```python
from build123d import *

# Parameters (mm, degrees)
SKETCH_W             = 140
SKETCH_H             = 102
PAD_DEPTH            = 30
SKETCH001_W          = 56.560638
SKETCH001_H          = 58.617586
SKETCH001_W_2        = 18.878723
SKETCH001_W_3        = 44
SKETCH001_H_2        = 35.382414
POCKET_DEPTH         = 28
FILLET_R             = 5
SKETCH002_W          = 65
SKETCH002_H          = 90
POCKET001_DEPTH      = 8
FILLET001_R          = 2
BODY_PLACEMENT_ANGLE = 90


with BuildPart() as part:
    # Sketch → Pad (new body)
    with BuildSketch(Plane.XY):
        Rectangle(SKETCH_W, SKETCH_H)
    extrude(amount=PAD_DEPTH)

    # Sketch001 (on DatumPlane) → Pocket (cut)
    with BuildSketch(Plane.XY.offset(30)):
        with Locations((-39.719681, 18.691207)):
            Rectangle(SKETCH001_W, SKETCH001_H)
        with Locations((18.840958, 18.691207)):
            Rectangle(SKETCH001_W, SKETCH001_H)
        with Locations((58.560638, 18.691207)):
            Rectangle(SKETCH001_W_2, SKETCH001_H)
        with Locations((-46, -30.308793)):
            Rectangle(SKETCH001_W_3, SKETCH001_H_2)
        with Locations((0, -30.308793)):
            Rectangle(SKETCH001_W_3, SKETCH001_H_2)
        with Locations((46, -30.308793)):
            Rectangle(SKETCH001_W_3, SKETCH001_H_2)
    extrude(amount=-POCKET_DEPTH, mode=Mode.SUBTRACT)

    # Fillet
    fillet_edges = [part.edges().sort_by_distance(p)[0] for p in [
        (-46, -12.617586, 2),
        (-24, -30.308793, 2),
        (-46, -48, 2),
        (-68, -30.308793, 2),
        (-39.719681, 48, 2),
        (-11.439362, 18.691207, 2),
        (-39.719681, -10.617586, 2),
        (-68, 18.691207, 2),
        (18.840958, 48, 2),
        (47.121277, 18.691207, 2),
        (18.840958, -10.617586, 2),
        (-9.439361, 18.691207, 2),
        (0, -12.617586, 2),
        (22, -30.308793, 2),
        (0, -48, 2),
        (-22, -30.308793, 2),
        (46, -12.617586, 2),
        (68, -30.308793, 2),
        (46, -48, 2),
        (24, -30.308793, 2),
        (58.560638, 48, 2),
        (68, 18.691207, 2),
        (58.560638, -10.617586, 2),
        (49.121277, 18.691207, 2),
    ]]
    fillet(fillet_edges, radius=FILLET_R)

    # Sketch002 (on DatumPlane) → Pocket001 (cut)
    with BuildSketch(Plane.XY.offset(30)):
        with Locations((-34.5, 0)):
            Rectangle(SKETCH002_W, SKETCH002_H)
        with Locations((34.5, 0)):
            Rectangle(SKETCH002_W, SKETCH002_H)
    extrude(amount=-POCKET001_DEPTH, mode=Mode.SUBTRACT)

    # Fillet001
    fillet001_edges = [part.edges().sort_by_distance(p)[0] for p in [
        (0, 51, 0),
        (70, 0, 0),
        (0, -51, 0),
        (-70, 0, 0),
    ]]
    fillet(fillet001_edges, radius=FILLET001_R)


with BuildPart() as part_1:
    # Body placement: moved
    add(part.part.moved(Location((151, 90, 0))).rotate(Axis((151, 90, 0), (0, 0, 1)), BODY_PLACEMENT_ANGLE))


solid = part_1.part
```
Part model, mm, in its own coordinate system. Round coordinates to 2 decimals unless told otherwise and drop trailing zeros. Write each loop counter-clockwise with the first axis right and the second up, starting at its lowest first coordinate (ties: lowest second). Pieces come first, ordered by that corner, then holes.
Item 1: Two-plate mould, pull along Y, no slides. Class faces 1 (the flat face through (182, 158, 19)), 2 (the flat face through (105, 79, 30)): +Y half, -Y half, draft (parallel to the pull), parting line (faces both ways), or undercut.
Results:
face 1: undercut
face 2: draft
Item 2: Cut at D-D, the plane y = 124. Give the cut face in (x, z).
Results:
outline: (100, 2) arc R2 ccw to (102, 0) - (200, 0) arc R2 ccw to (202, 2) - (202, 30) - (199, 30) - (199, 7) arc R5 cw to (194, 2) - (168.62, 2) arc R5 cw to (163.62, 7) - (163.62, 22) - (161.62, 22) - (161.62, 7) arc R5 cw to (156.62, 2) - (108, 2) arc R5 cw to (103, 7) - (103, 30) - (100, 30) - close
Item 3: Probe L1, parallel to X at y = 126, z = 14.25; L2, parallel to Y at x = 195, z = 10; L3, parallel to Y at x = 117, z = 8.5. List the from-to ranges inside material, lowest first.
Results:
L1: x = 100 to 103, 161.62 to 163.62, 199 to 202
L2: y = 20 to 22, 66 to 68, 112 to 114, 158 to 160
L3: y = 20 to 22, 78.56 to 80.56, 137.12 to 139.12, 158 to 160
Item 4: Cut at B-B, the plane x = 121. Give the cut face in (y, z), plus the area to 3 significant figures.
Results:
outline: (20, 2) arc R2 ccw to (22, 0) - (158, 0) arc R2 ccw to (160, 2) - (160, 30) - (158, 30) - (158, 7) arc R5 cw to (153, 2) - (144.12, 2) arc R5 cw to (139.12, 7) - (139.12, 22) - (137.12, 22) - (137.12, 7) arc R5 cw to (132.12, 2) - (85.56, 2) arc R5 cw to (80.56, 7) - (80.56, 22) - (78.56, 22) - (78.56, 7) arc R5 cw to (73.56, 2) - (27, 2) arc R5 cw to (22, 7) - (22, 30) - (20, 30) - close
area: 502 mm2
Item 5: Cut at A-A, the plane z = 8.5. Give the cut face in (x, y), plus the area to 3 significant figures.
Results:
outline: (100, 20) - (202, 20) - (202, 160) - (100, 160) - close; hole (103, 22) - (161.62, 22) - (161.62, 78.56) - (103, 78.56) - close; hole (103, 80.56) - (161.62, 80.56) - (161.62, 137.12) - (103, 137.12) - close; hole (103, 139.12) - (161.62, 139.12) - (161.62, 158) - (103, 158) - close; hole (163.62, 22) - (199, 22) - (199, 66) - (163.62, 66) - close; hole (163.62, 68) - (199, 68) - (199, 112) - (163.62, 112) - close; hole (163.62, 114) - (199, 114) - (199, 158) - (163.62, 158) - close
area: 1,870 mm2
Item 6: Cut at C-C, the plane z = 24.75. Count the separate pieces of the cut face and the enclosed holes in it, plus the area to 3 significant figures.
Results:
separate pieces: 2
enclosed holes: 1
area: 1,260 mm2
Item 7: Drop a flat-ended pin along its axis: pin 1 Ø7 at (x, y) = (136, 150) entering from +Z. Give the stop position or say it passes through.
Results:
pin 1: stops at z = 2.03
